Job drawing, mm, ordinate dimensions from the low corner. One solid piece. A direction names the side the tool comes from. Give positions to 0.01 mm unless a question says otherwise; leave off trailing zeros. Order: outer loops, then holes, each group sorted by start corner. A loop starts at its lowest first (then second) coordinate and runs counter-clockwise, first axis right, second up. Notation, with made-up numbers: (78.5, 4.25) -> (88.5, 4.25) arc R33 ccw to (88.5, 41.25) -> close; hole circle Ø7 at (30.5, -28). An arc over 180 degrees is marked (long way). Use CSV: the item, a comma, the result in double quotes. Start each with the question number.
1. Cut at B-B on x = 44. List the corners of the cut face in (y, z).
2. Cut at A-A on y = 30.5. List the corners of the cut face in (x, z).
3. Cut at C-C on z = 3.25. List the corners of the cut face in (x, y).
4. Drop flat-ended pins along their axis: pin 1 (3 mm diameter, centred on x = 26.5, z = 7.5, fed in from +Y); pin 2 (4 mm diameter, centred on y = 29, z = 1.5, fed in from +X); pin 3 (3.5 mm diameter, centred on x = 26.5, z = 5, fed in from -Y); pin 4 (12 mm diameter, centred on x = 38.5, y = 25.5, fed in from -Z). Give the stop position or say it passes through.
5. 3-axis set-ups, long thin cutter, end or side, ignore diameter. For the marked faces 5, 6, 7 and 8: which of +Z, -Z, +X, -X, +Y, -Y reach the whole face in a straight line?
6. Cut at D-D on x = 8.25. List the corners of the cut face in (y, z).
7. Pull direction X, two halves, no side cores. Call the marked faces 1, 2, 3 and 4: released by +X, released by -X, zero draft, split by the parting line, or undercut.
8. Wall check: line 1 (Y direction, x = 8.25, z = 2.1); line 2 (Y direction, x = 29.5, z = 5.5); line 3 (X direction, y = 14, z = 1). Give the ranges that are in metal, low to high. Write a range as from..to.
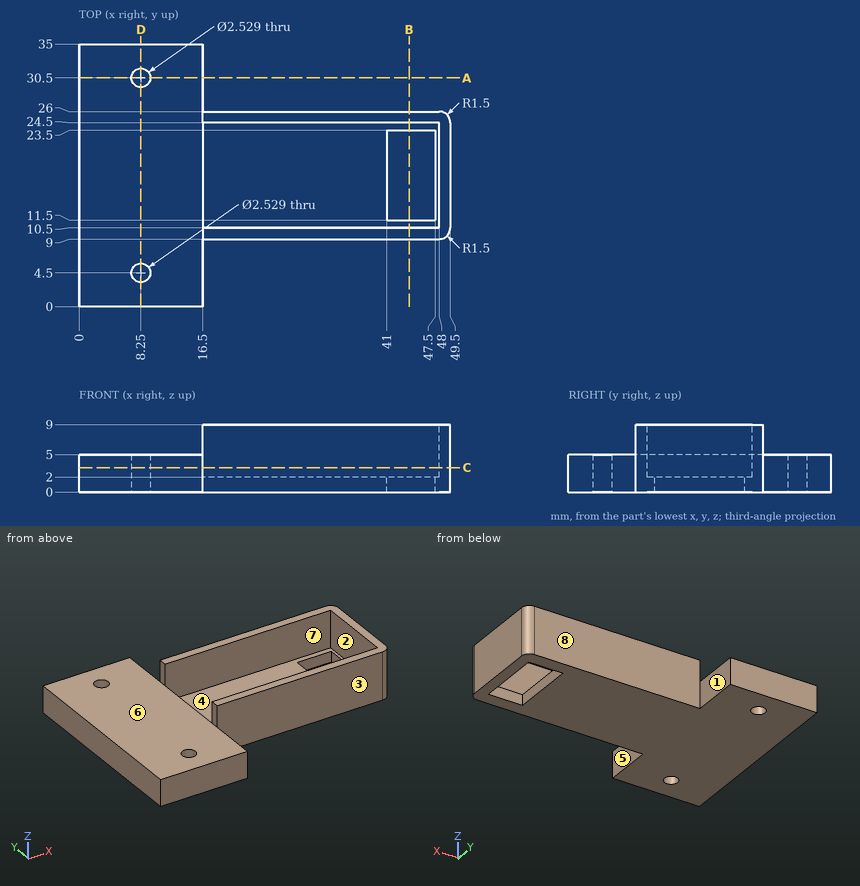
Verdict:
1,outline,"(9, 0) -> (11.5, 0) -> (11.5, 2) -> (10.5, 2) -> (10.5, 9) -> (9, 9) -> close; (23.5, 0) -> (26, 0) -> (26, 9) -> (24.5, 9) -> (24.5, 2) -> (23.5, 2) -> close"
2,outline,"(0, 0) -> (6.99, 0) -> (6.99, 5) -> (0, 5) -> close; (9.51, 0) -> (16.5, 0) -> (16.5, 5) -> (9.51, 5) -> close"
3,outline,"(0, 0) -> (16.5, 0) -> (16.5, 9) -> (48, 9) arc R1.5 ccw to (49.5, 10.5) -> (49.5, 24.5) arc R1.5 ccw to (48, 26) -> (16.5, 26) -> (16.5, 35) -> (0, 35) -> close; hole circle Ø2.53 at (8.25, 4.5); hole circle Ø2.53 at (8.25, 30.5); hole (16.5, 10.5) -> (48, 10.5) -> (48, 24.5) -> (16.5, 24.5) -> close"
4,pin 1,"y = 26"
4,pin 2,"x = 16.5"
4,pin 3,"y = 9"
4,pin 4,"z = 0"
5,face 5,"+Z, -Z, +X, -Y"
5,face 6,"+Z, -X, +Y, -Y"
5,face 7,"+Z"
5,face 8,"+Z, -Z, +X, +Y"
6,outline,"(0, 0) -> (3.24, 0) -> (3.24, 5) -> (0, 5) -> close; (5.76, 0) -> (29.24, 0) -> (29.24, 5) -> (5.76, 5) -> close; (31.76, 0) -> (35, 0) -> (35, 5) -> (31.76, 5) -> close"
7,face 1,"released by +X"
7,face 2,"undercut"
7,face 3,"zero draft"
7,face 4,"undercut"
8,line 1,"0..3.24, 5.76..29.24, 31.76..35"
8,line 2,"9..10.5, 24.5..26"
8,line 3,"0..41, 47.5..49.5"
